The model under review builds one solid part; all positions refer to its coordinate system, in mm. A direction names the side the tool comes from. Coordinates: 2 decimals unless noted, no trailing zeros. Write each loop counter-clockwise with the first axis right and the second up, starting at its lowest first coordinate (ties: lowest second). Pieces come first, ordered by that corner, then holes. Notation, with made-up numbers: (-15.75, 69.5) -> (41.25, 69.5) arc R23 ccw to (41.25, 78.5) -> close; hole circle Ø6 at (20.25, -1.75). An arc over 180 degrees is marked (long way). Write each question's results on one line, items separated by ' | '.
```python
from build123d import *

# Parameters (mm, degrees)
SKETCH1_R           = 5
BOSS_EXTRUDE1_DEPTH = 25
CUT_EXTRUDE1_DEPTH  = 8
BOSS_EXTRUDE2_DEPTH = 10
SKETCH4_W           = 5.15
SKETCH4_H           = 5.15
CUT_EXTRUDE2_DEPTH  = 10
FILLET1_R           = 0.5


with BuildPart() as part:
    # Sketch1 → Boss-Extrude1 (new body)
    with BuildSketch(Plane.XY):
        Circle(SKETCH1_R)
    extrude(amount=BOSS_EXTRUDE1_DEPTH)

    # Sketch2 → Cut-Extrude1 (cut)
    with BuildSketch(Plane(origin=(0, 0, 0), x_dir=(-1, 0, 0), z_dir=(0, 0, -1))):
        with BuildLine():
            Line((-2.221320345, -1.785563195), (2.221320345, -1.785563195))
            ThreePointArc((2.221320345, -1.785563195), (2.849942511, 0.018102015), (2.198459265, 1.813636364))
            Line((2.198459265, 1.813636364), (-2.198459265, 1.813636364))
            ThreePointArc((-2.198459265, 1.813636364), (-2.849942511, 0.018102015), (-2.221320345, -1.785563195))
        make_face()
    extrude(amount=-CUT_EXTRUDE1_DEPTH, mode=Mode.SUBTRACT)

    # Sketch3 → Boss-Extrude2 (add)
    with BuildSketch(Plane.XY.offset(25)):
        with BuildLine():
            ThreePointArc((-4, -3), (-3.535533906, -3.535533906), (-3, -4))
            Line((-3, -4), (3, -4))
            ThreePointArc((3, -4), (3.535533906, -3.535533906), (4, -3))
            Line((4, -3), (4, 3))
            ThreePointArc((4, 3), (3.535533906, 3.535533906), (3, 4))
            Line((3, 4), (-3, 4))
            ThreePointArc((-3, 4), (-3.535533906, 3.535533906), (-4, 3))
            Line((-4, 3), (-4, -3))
        make_face()
    extrude(amount=BOSS_EXTRUDE2_DEPTH)

    # Sketch4 → Cut-Extrude2 (cut)
    with BuildSketch(Plane.XY.offset(35)):
        Rectangle(SKETCH4_W, SKETCH4_H)
    extrude(amount=-CUT_EXTRUDE2_DEPTH, mode=Mode.SUBTRACT)

    # Fillet1
    fillet1_edges = [part.edges().sort_by_distance(p)[0] for p in [
        (-5, 0, 0),
    ]]
    fillet(fillet1_edges, radius=FILLET1_R)


solid = part.part
```
Q1. Clearance check with flat-ended pins moving along their axes: P1, Ø1.5, axis at y = 0.5, z = 29, coming from the +X side; P2, Ø4, axis at x = -3.5, z = 19, coming from the +Y side; P3, Ø2, axis at y = 2, z = 13, coming from the +X side. State where each tip first meets the part, or that it passes through.
Solution:
P1: x = 4 | P2: y = 4.77 | P3: x = 4.9
Q2. Add section B-B (y = 0). Write out the cut boundary in (x, z) (3 decimals).
Solution:
outline: (-5, 0.5) arc R0.5 ccw to (-4.5, 0) -> (-2.85, 0) -> (-2.85, 8) -> (2.85, 8) -> (2.85, 0) -> (4.5, 0) arc R0.5 ccw to (5, 0.5) -> (5, 25) -> (4, 25) -> (4, 35) -> (2.575, 35) -> (2.575, 25) -> (-2.575, 25) -> (-2.575, 35) -> (-4, 35) -> (-4, 25) -> (-5, 25) -> close
Q3. Draft analysis for pull direction Y (two halves, no side actions). For faces 4 (the cylindrical face through (-2.85, -0.01, 3.94)), 5 (the flat face through (2.575, 0, 30)), 6 (the flat face through (0, -2, 0)), 7 (the flat face through (0, 4, 30)), state which applies: pulls with the +Y half, pulls with the -Y half, needs draft (parallel to the pull), parting line crosses it, or undercut.
Solution:
face 4: undercut | face 5: undercut | face 6: needs draft | face 7: pulls with the +Y half
Q4. For line 1 (Y direction, x = -1.25, z = 26) (3 decimals); line 2 (Y direction, x = 3, z = 25); line 3 (Z direction, x = -2.75, y = 0), list the stretches that pass through material, from the lowest coordinate up. Write a range as from..to.
Solution:
line 1: -4..-2.575, 2.575..4 | line 2: -4..4 | line 3: 8..35
Q5. Add section D-D (z = 7). Write out the cut boundary in (x, y).
Solution:
outline: circle Ø10 at (0, 0); hole (-2.22, -1.79) -> (2.22, -1.79) arc R2.85 ccw to (2.2, 1.81) -> (-2.2, 1.81) arc R2.85 ccw to start
Q6. Machinability: for faces 1 (the cylindrical face through (2.85, 0.05, 3.94)), 2 (the flat face through (0, -4.4, 25)), 3 (the flat face through (0, 2.575, 30)), which of the approach directions +Z, -Z, +X, -X, +Y, -Y give a long, thin tool a straight path to every point of the face, cutting with its end or side? Answer none if there is none.
Solution:
face 1: -Z | face 2: +Z, +X, -X, -Y | face 3: +Z
Q7. Add section C-C (x = 0). Write out the cut boundary in (y, z) (3 decimals).
Solution:
outline: (-5, 0.5) arc R0.5 ccw to (-4.5, 0) -> (-1.786, 0) -> (-1.786, 8) -> (1.814, 8) -> (1.814, 0) -> (4.5, 0) arc R0.5 ccw to (5, 0.5) -> (5, 25) -> (4, 25) -> (4, 35) -> (2.575, 35) -> (2.575, 25) -> (-2.575, 25) -> (-2.575, 35) -> (-4, 35) -> (-4, 25) -> (-5, 25) -> close
Q8. Add section A-A (z = 33). Write out the cut boundary in (x, y) (3 decimals).
Solution:
outline: (-4, -3) arc R5 ccw to (-3, -4) -> (3, -4) arc R5 ccw to (4, -3) -> (4, 3) arc R5 ccw to (3, 4) -> (-3, 4) arc R5 ccw to (-4, 3) -> close; hole (-2.575, -2.575) -> (2.575, -2.575) -> (2.575, 2.575) -> (-2.575, 2.575) -> close
